CAD build for the part. Positions are in the model's coordinates, mm. A direction names the side the tool comes from. Give positions to 0.01 mm unless a question says otherwise; leave off trailing zeros. Loops run counter-clockwise (first coordinate to the right, second up) from the corner with the lowest first, then second, coordinate; pieces in that order, holes last. Notation, with made-up numbers: (-14, 52) -> (19, 52) arc R3 cw to (19, 56) -> close; hole circle Ø9 at (76, -24.75). An arc over 180 degrees is marked (long way). Write each question's results on one line, items separated by ' | '. Start each with the question number.
```python
from build123d import *

# Parameters (mm, degrees)
CROQUIS1_R              = 8.15
CROQUIS1_R_2            = 1.6
SALIENTE_EXTRUIR1_DEPTH = 5
CROQUIS2_R              = 9.1
CORTAR_EXTRUIR1_DEPTH   = 1
CORTAR_EXTRUIR2_DEPTH   = 3
REDONDEO1_R             = 1
SALIENTE_EXTRUIR2_DEPTH = 46
CORTAR_EXTRUIR3_DEPTH   = 2
CORTAR_EXTRUIR4_REACH   = 103.242
CROQUIS6_R              = 2.6
CROQUIS6_W              = 5.6
CROQUIS6_H              = 3
CORTAR_EXTRUIR5_DEPTH   = 5
SALIENTE_EXTRUIR3_DEPTH = 46
CORTAR_EXTRUIR6_DEPTH   = 2
CORTAR_EXTRUIR7_REACH   = 103.242
CROQUIS10_R             = 2.6
CROQUIS10_W             = 5.6
CROQUIS10_H             = 3
CROQUIS11_R             = 1.6
CORTAR_EXTRUIR8_DEPTH   = 21
REDONDEO2_R             = 1


with BuildPart() as part:
    # Croquis1 → Saliente-Extruir1 (new body)
    with BuildSketch(Plane(origin=(0, 0, 0), x_dir=(1, 0, 0), z_dir=(0, 1, 0))):
        with BuildLine():
            Line((-30, -35), (30, -35))
            ThreePointArc((30, -35), (47.67766953, -27.67766953), (55, -10))
            Line((55, -10), (55, 15))
            ThreePointArc((55, 15), (49.142135624, 29.142135624), (35, 35))
            Line((35, 35), (-35, 35))
            ThreePointArc((-35, 35), (-49.142135624, 29.142135624), (-55, 15))
            Line((-55, 15), (-55, -10))
            ThreePointArc((-55, -10), (-47.67766953, -27.67766953), (-30, -35))
        make_face()
        with Locations(Location((39, 9, 0), (0, 0, 270))):
            Circle(CROQUIS1_R, mode=Mode.SUBTRACT)
        with Locations(Location((51.75, 12, 0), (0, 0, 270))):
            Circle(CROQUIS1_R_2, mode=Mode.SUBTRACT)
        with Locations(Location((-39, 9, 0), (0, 0, 90))):
            Circle(CROQUIS1_R, mode=Mode.SUBTRACT)
        with Locations(Location((51.75, -7, 0), (0, 0, 90))):
            Circle(CROQUIS1_R_2, mode=Mode.SUBTRACT)
        with Locations(Location((-51.75, -7, 0), (0, 0, 270))):
            Circle(CROQUIS1_R_2, mode=Mode.SUBTRACT)
        with Locations(Location((-51.75, 12, 0), (0, 0, 90))):
            Circle(CROQUIS1_R_2, mode=Mode.SUBTRACT)
        with BuildLine():
            Line((-10, -23), (10, -23))
            ThreePointArc((10, -23), (17.071067812, -20.071067812), (20, -13))
            Line((20, -13), (20, 13))
            ThreePointArc((20, 13), (17.071067812, 20.071067812), (10, 23))
            Line((10, 23), (-10, 23))
            ThreePointArc((-10, 23), (-17.071067812, 20.071067812), (-20, 13))
            Line((-20, 13), (-20, -13))
            ThreePointArc((-20, -13), (-17.071067812, -20.071067812), (-10, -23))
        make_face(mode=Mode.SUBTRACT)
    extrude(amount=SALIENTE_EXTRUIR1_DEPTH)

    # Croquis2 → Cortar-Extruir1 (cut)
    with BuildSketch(Plane(origin=(0, 5, 0), x_dir=(1, 0, 0), z_dir=(0, 1, 0))):
        with Locations(Location((39, 9, 0), (0, 0, 270))):
            Circle(CROQUIS2_R)
        with Locations(Location((-39, 9, 0), (0, 0, 90))):
            Circle(CROQUIS2_R)
    extrude(amount=-CORTAR_EXTRUIR1_DEPTH, mode=Mode.SUBTRACT)

    # Croquis3 → Cortar-Extruir2 (cut)
    with BuildSketch(Plane(origin=(0, 5, 0), x_dir=(1, 0, 0), z_dir=(0, 1, 0))):
        with BuildLine():
            Line((51.75, 15), (55, 15))
            Line((55, 15), (55, 9))
            Line((55, 9), (51.75, 9))
            ThreePointArc((51.75, 9), (48.75, 12), (51.75, 15))
        make_face()
        with BuildLine():
            Line((51.75, -10), (55, -10))
            Line((55, -10), (55, -4))
            Line((55, -4), (51.75, -4))
            ThreePointArc((51.75, -4), (48.75, -7), (51.75, -10))
        make_face()
        with BuildLine():
            Line((-51.75, -4), (-55, -4))
            Line((-55, -4), (-55, -10))
            Line((-55, -10), (-51.75, -10))
            ThreePointArc((-51.75, -10), (-48.75, -7), (-51.75, -4))
        make_face()
        with BuildLine():
            Line((-51.75, 15), (-55, 15))
            Line((-55, 15), (-55, 9))
            Line((-55, 9), (-51.75, 9))
            ThreePointArc((-51.75, 9), (-48.75, 12), (-51.75, 15))
        make_face()
    extrude(amount=-CORTAR_EXTRUIR2_DEPTH, mode=Mode.SUBTRACT)

    # Redondeo1
    redondeo1_edges = [part.edges().sort_by_distance(p)[0] for p in [
        (-55, 3.5, -9),
        (-55, 3.5, 4),
        (55, 3.5, 4),
        (55, 3.5, -9),
        (55, 3.5, -15),
        (55, 3.5, 10),
        (-55, 3.5, 10),
        (-55, 3.5, -15),
    ]]
    fillet(redondeo1_edges, radius=REDONDEO1_R)

    # Croquis4 → Saliente-Extruir2 (add)
    with BuildSketch(Plane(origin=(0, 5, 0), x_dir=(1, 0, 0), z_dir=(0, 1, 0))):
        with BuildLine():
            Line((-25, 35), (25, 35))
            Line((25, 35), (25, 28))
            ThreePointArc((25, 28), (23.535533906, 24.464466094), (20, 23))
            Line((20, 23), (-20, 23))
            ThreePointArc((-20, 23), (-23.535533906, 24.464466094), (-25, 28))
            Line((-25, 28), (-25, 35))
        make_face()
    extrude(amount=SALIENTE_EXTRUIR2_DEPTH)

    # Croquis5 → Cortar-Extruir3 (cut)
    with BuildSketch(Plane(origin=(0, 0, -35), x_dir=(-1, 0, 0), z_dir=(0, 0, -1))):
        with BuildLine():
            Line((-25, 51), (25, 51))
            Line((25, 51), (25, 17.708712153))
            ThreePointArc((25, 17.708712153), (22.970514841, 15.371172764), (20, 14.5))
            Line((20, 14.5), (-20, 14.5))
            ThreePointArc((-20, 14.5), (-22.970514841, 15.371172764), (-25, 17.708712153))
            Line((-25, 17.708712153), (-25, 51))
        make_face()
    extrude(amount=-CORTAR_EXTRUIR3_DEPTH, mode=Mode.SUBTRACT)

    # Cortar-Extruir4: up to this face of the body (flat: up to its plane)
    cortar_extruir4_end = Plane(part.part.faces().sort_by_distance((0, 26.68556701, -23))[0])
    # Croquis6 → Cortar-Extruir4 (cut, up to the picked face)
    with BuildSketch(Plane(origin=(0, 0, -33), x_dir=(-1, 0, 0), z_dir=(0, 0, -1)), mode=Mode.PRIVATE) as cortar_extruir4_sk1:
        with Locations((-20, 20)):
            Circle(CROQUIS6_R)
    cortar_extruir4_tool1 = split(extrude(cortar_extruir4_sk1.sketch, amount=-CORTAR_EXTRUIR4_REACH, mode=Mode.PRIVATE), bisect_by=cortar_extruir4_end, keep=Keep.BOTH, mode=Mode.PRIVATE)
    # Croquis6 → Cortar-Extruir4 (cut, up to the picked face)
    with BuildSketch(Plane(origin=(0, 0, -33), x_dir=(-1, 0, 0), z_dir=(0, 0, -1)), mode=Mode.PRIVATE) as cortar_extruir4_sk2:
        with Locations(Location((20, 20, 0), (0, 0, 90))):
            Circle(CROQUIS6_R)
    cortar_extruir4_tool2 = split(extrude(cortar_extruir4_sk2.sketch, amount=-CORTAR_EXTRUIR4_REACH, mode=Mode.PRIVATE), bisect_by=cortar_extruir4_end, keep=Keep.BOTH, mode=Mode.PRIVATE)
    # Croquis6 → Cortar-Extruir4 (cut, up to the picked face)
    with BuildSketch(Plane(origin=(0, 0, -33), x_dir=(-1, 0, 0), z_dir=(0, 0, -1)), mode=Mode.PRIVATE) as cortar_extruir4_sk3:
        with Locations((-20, 44.5)):
            Rectangle(CROQUIS6_W, CROQUIS6_H)
    cortar_extruir4_tool3 = split(extrude(cortar_extruir4_sk3.sketch, amount=-CORTAR_EXTRUIR4_REACH, mode=Mode.PRIVATE), bisect_by=cortar_extruir4_end, keep=Keep.BOTH, mode=Mode.PRIVATE)
    # Croquis6 → Cortar-Extruir4 (cut, up to the picked face)
    with BuildSketch(Plane(origin=(0, 0, -33), x_dir=(-1, 0, 0), z_dir=(0, 0, -1)), mode=Mode.PRIVATE) as cortar_extruir4_sk4:
        with Locations((20, 44.5)):
            Rectangle(CROQUIS6_W, CROQUIS6_H)
    cortar_extruir4_tool4 = split(extrude(cortar_extruir4_sk4.sketch, amount=-CORTAR_EXTRUIR4_REACH, mode=Mode.PRIVATE), bisect_by=cortar_extruir4_end, keep=Keep.BOTH, mode=Mode.PRIVATE)
    add(cortar_extruir4_tool1.solids().sort_by(Axis((20, 20, -33), (0, 0, 1)))[0], mode=Mode.SUBTRACT)
    add(cortar_extruir4_tool2.solids().sort_by(Axis((-20, 20, -33), (0, 0, 1)))[0], mode=Mode.SUBTRACT)
    add(cortar_extruir4_tool3.solids().sort_by(Axis((20, 44.5, -33), (0, 0, 1)))[0], mode=Mode.SUBTRACT)
    add(cortar_extruir4_tool4.solids().sort_by(Axis((-20, 44.5, -33), (0, 0, 1)))[0], mode=Mode.SUBTRACT)

    # Croquis7 → Cortar-Extruir5 (cut)
    with BuildSketch(Plane.XY.offset(-23)):
        Polygon((-20, 24.7), (-24.070319398, 22.35), (-24.070319398, 17.65), (-20, 15.3), (-15.929680602, 17.65), (-15.929680602, 22.35), align=None)
        Polygon((15.929680602, 22.35), (20, 24.7), (24.070319398, 22.35), (24.070319398, 17.65), (20, 15.3), (15.929680602, 17.65), align=None)
    extrude(amount=-CORTAR_EXTRUIR5_DEPTH, mode=Mode.SUBTRACT)

    # Croquis8 → Saliente-Extruir3 (add)
    with BuildSketch(Plane(origin=(0, 5, 0), x_dir=(1, 0, 0), z_dir=(0, 1, 0))):
        with BuildLine():
            Line((-10, -35), (10, -35))
            Line((10, -35), (10, -28))
            ThreePointArc((10, -28), (8.535533906, -24.464466094), (5, -23))
            Line((5, -23), (-5, -23))
            ThreePointArc((-5, -23), (-8.535533906, -24.464466094), (-10, -28))
            Line((-10, -28), (-10, -35))
        make_face()
    extrude(amount=SALIENTE_EXTRUIR3_DEPTH)

    # Croquis9 → Cortar-Extruir6 (cut)
    with BuildSketch(Plane.XY.offset(35)):
        with BuildLine():
            Line((10, 17.708712153), (10, 51))
            Line((10, 51), (-10, 51))
            Line((-10, 51), (-10, 17.708712153))
            ThreePointArc((-10, 17.708712153), (-7.970514841, 15.371172764), (-5, 14.5))
            Line((-5, 14.5), (5, 14.5))
            ThreePointArc((5, 14.5), (7.970514841, 15.371172764), (10, 17.708712153))
        make_face()
    extrude(amount=-CORTAR_EXTRUIR6_DEPTH, mode=Mode.SUBTRACT)

    # Cortar-Extruir7: up to this face of the body (flat: up to its plane)
    cortar_extruir7_end = Plane(part.part.faces().sort_by_distance((0, 23.446428571, 23))[0])
    # Croquis10 → Cortar-Extruir7 (cut, up to the picked face)
    with BuildSketch(Plane.XY.offset(33), mode=Mode.PRIVATE) as cortar_extruir7_sk1:
        with Locations((-5, 20)):
            Circle(CROQUIS10_R)
    cortar_extruir7_tool1 = split(extrude(cortar_extruir7_sk1.sketch, amount=-CORTAR_EXTRUIR7_REACH, mode=Mode.PRIVATE), bisect_by=cortar_extruir7_end, keep=Keep.BOTH, mode=Mode.PRIVATE)
    # Croquis10 → Cortar-Extruir7 (cut, up to the picked face)
    with BuildSketch(Plane.XY.offset(33), mode=Mode.PRIVATE) as cortar_extruir7_sk2:
        with Locations(Location((5, 20, 0), (0, 0, 90))):
            Circle(CROQUIS10_R)
    cortar_extruir7_tool2 = split(extrude(cortar_extruir7_sk2.sketch, amount=-CORTAR_EXTRUIR7_REACH, mode=Mode.PRIVATE), bisect_by=cortar_extruir7_end, keep=Keep.BOTH, mode=Mode.PRIVATE)
    # Croquis10 → Cortar-Extruir7 (cut, up to the picked face)
    with BuildSketch(Plane.XY.offset(33), mode=Mode.PRIVATE) as cortar_extruir7_sk3:
        with Locations((-5, 44.5)):
            Rectangle(CROQUIS10_W, CROQUIS10_H)
    cortar_extruir7_tool3 = split(extrude(cortar_extruir7_sk3.sketch, amount=-CORTAR_EXTRUIR7_REACH, mode=Mode.PRIVATE), bisect_by=cortar_extruir7_end, keep=Keep.BOTH, mode=Mode.PRIVATE)
    # Croquis10 → Cortar-Extruir7 (cut, up to the picked face)
    with BuildSketch(Plane.XY.offset(33), mode=Mode.PRIVATE) as cortar_extruir7_sk4:
        with Locations((5, 44.5)):
            Rectangle(CROQUIS10_W, CROQUIS10_H)
    cortar_extruir7_tool4 = split(extrude(cortar_extruir7_sk4.sketch, amount=-CORTAR_EXTRUIR7_REACH, mode=Mode.PRIVATE), bisect_by=cortar_extruir7_end, keep=Keep.BOTH, mode=Mode.PRIVATE)
    add(cortar_extruir7_tool1.solids().sort_by(Axis((-5, 20, 33), (0, 0, -1)))[0], mode=Mode.SUBTRACT)
    add(cortar_extruir7_tool2.solids().sort_by(Axis((5, 20, 33), (0, 0, -1)))[0], mode=Mode.SUBTRACT)
    add(cortar_extruir7_tool3.solids().sort_by(Axis((-5, 44.5, 33), (0, 0, -1)))[0], mode=Mode.SUBTRACT)
    add(cortar_extruir7_tool4.solids().sort_by(Axis((5, 44.5, 33), (0, 0, -1)))[0], mode=Mode.SUBTRACT)

    # Croquis11 → Cortar-Extruir8 (cut)
    with BuildSketch(Plane(origin=(0, 51, 0), x_dir=(1, 0, 0), z_dir=(0, 1, 0))):
        with Locations(Location((-5, -28, 0), (0, 0, 270))):
            Circle(CROQUIS11_R)
        with Locations(Location((-20, 28, 0), (0, 0, 270))):
            Circle(CROQUIS11_R)
        with Locations(Location((5, -28, 0), (0, 0, 270))):
            Circle(CROQUIS11_R)
        with Locations(Location((20, 28, 0), (0, 0, 270))):
            Circle(CROQUIS11_R)
    extrude(amount=-CORTAR_EXTRUIR8_DEPTH, mode=Mode.SUBTRACT)

    # Redondeo2
    redondeo2_edges = [part.edges().sort_by_distance(p)[0] for p in [
        (25, 17.708712153, -34),
        (-25, 17.708712153, -34),
        (10, 17.708712153, 34),
        (-10, 17.708712153, 34),
    ]]
    fillet(redondeo2_edges, radius=REDONDEO2_R)


solid = part.part
```
Q1. Mould opens along Z. For faces 4 (the face through (4.03, 48.54, 26.73)), 5 (the face through (-22.01, 23.54, -25.46)), 6 (the face through (0, 33, -33)) say: pulls with the +Z half, pulls with the -Z half, needs draft (parallel to the pull), parting line crosses it, or undercut.
Q2. Saw through at A-A, the plane y = 47.5. List the corners of the cut face in (x, z), then the cut area to 3 significant figures.
Q3. Saw through at B-B, the plane z = 7. List the corners of the cut face in (x, y), then the cut area to 3 significant figures.
Q4. Saw through at C-C, the plane x = -36.5. List the corners of the cut face in (y, z), then the cut area to 3 significant figures.
Q5. Wall check: L1, parallel to X at y = 32.5, z = 28; L2, parallel to X at y = 36, z = -28; L3, parallel to Z at x = -51.75, y = 1.15. Give the ranges that are in metal, low to high.
Q6. Drop flat-ended pins along their axis: pin 1 (8 mm diameter, centred on y = 14.5, z = -27, fed in from +X); pin 2 (12 mm diameter, centred on y = 21, z = 25.5, fed in from +X); pin 3 (4 mm diameter, centred on x = 5, z = 28, fed in from -Y); pin 4 (3.5 mm diameter, centred on x = -51.75, z = 7, fed in from +Y). Give the stop position or say it passes through.
Q7. Which spindle directions (+Z, -Z, +X, -X, +Y, -Y) get a long thin tool onto all of the face, cutting with end or side? Do faces 1 (the face through (-17.15, 2.46, 19.99)), 2 (the face through (53, 4, -9)), 3 (the face through (-2.2, 44, 28)). Say none if no direction does.
Answer block:
1) face 4: undercut | face 5: needs draft | face 6: pulls with the -Z half
2) outline: (-25, -33) -> (25, -33) -> (25, -28) arc R5 ccw to (20, -23) -> (-20, -23) arc R5 ccw to (-25, -28) -> close; (-10, 28) arc R5 ccw to (-5, 23) -> (5, 23) arc R5 ccw to (10, 28) -> (10, 33) -> (-10, 33) -> close; hole circle Ø3.2 at (-20, -28); hole circle Ø3.2 at (-5, 28); hole circle Ø3.2 at (5, 28); hole circle Ø3.2 at (20, -28) | area: 646 mm2
3) outline: (-55, 0) -> (-53.35, 0) -> (-53.35, 2) -> (-55, 2) -> close; (-50.15, 0) -> (-20, 0) -> (-20, 5) -> (-48.75, 5) -> (-48.75, 2) -> (-50.15, 2) -> close; (20, 0) -> (50.15, 0) -> (50.15, 2) -> (48.75, 2) -> (48.75, 5) -> (20, 5) -> close; (53.35, 0) -> (55, 0) -> (55, 2) -> (53.35, 2) -> close | area: 300 mm2
4) outline: (0, -34.94) -> (5, -34.94) -> (5, -17.75) -> (4, -17.75) -> (4, -16.76) -> (0, -16.76) -> close; (0, -1.24) -> (4, -1.24) -> (4, -0.25) -> (5, -0.25) -> (5, 34.14) -> (0, 34.14) -> close | area: 266 mm2
5) L1: x = -10 to -6.6, -3.4 to 3.4, 6.6 to 10 | L2: x = -25 to -21.6, -18.4 to 18.4, 21.6 to 25 | L3: z = -25.93 to -13.6, -10.4 to 5.4, 8.6 to 22.33
6) pin 1: stops at x = 25 | pin 2: stops at x = 10 | pin 3: stops at y = 0 | pin 4: stops at y = 2
7) face 1: +Y, -Y | face 2: +X, +Y | face 3: +Z
